Input: part model. Units: mm. Frame: model coordinates. A direction names the side the tool comes from. Round coordinates to 2 decimals unless told otherwise and drop trailing zeros. Order: outer loops, then holes, each group sorted by start corner. A loop starts at its lowest first (then second) coordinate and runs counter-clockwise, first axis right, second up.
Item 1: Cut plane C-C on y = 28.5. Output: boundary loops of the cut face in (x, z).
Item 2: Mould query, pull axis Y, two halves, no side actions, for faces 1 (the flat face through (95.14, 6.44, 33.84)), 2 (the cylindrical face through (9.68, 20.1, 3.13)), 3 (the flat face through (11.43, 7, -3)). Classes: released by +Y, released by -Y, zero draft, split by the parting line, or undercut.
Item 3: First-contact query: pin 1 (1.5 mm diameter, centred on x = 16.5, y = 26, fed in from +Z); pin 2 (6 mm diameter, centred on y = 13.5, z = 16.5, fed in from -X); pin 3 (1.5 mm diameter, centred on y = 8, z = -3, fed in from +X); pin 4 (6.5 mm diameter, centred on x = 51.816, z = -12.7, fed in from +Y). Flat tips, straight axial feed; report the tip coordinate or a pass-through.
Item 4: Cut plane A-A on z = -12.7. Output: boundary loops of the cut face in (x, y), then the cut area to 3 significant figures.
Item 5: Reachability of faces 4 (the flat face through (6, 13.97, -3)), 5 (the flat face through (38.1, 25, -13)), 6 (the flat face through (52, 25.4, -15)) from +Z, -Z, +X, -X, +Y, -Y: full face, straight path, thin tool, end or side. Return the list, or none.
Item 6: Line query: L1, parallel to Y at x = 6, z = 4; L2, parallel to X at y = 25.5, z = -12.5; L3, parallel to X at y = 20.5, z = -13. Output: solid intervals per line, ascending.
```python
from build123d import *

# Parameters (mm, degrees)
SKETCH2_R           = 2.0828
BOSS_EXTRUDE1_DEPTH = 31.75
SKETCH4_W           = 31.75
SKETCH4_H           = 12.7
CUT_EXTRUDE1_DEPTH  = 19.05
SKETCH5_R           = 3.4925
CUT_EXTRUDE2_DEPTH  = 6.35
CUT_EXTRUDE6_DEPTH  = 19.05
CHAMFER5_SIZE       = 12.7
CHAMFER7_SIZE       = 12.7
SKETCH6_R           = 3.4925
CUT_EXTRUDE8_DEPTH  = 25.4
SKETCH15_R          = 3.4925
SKETCH15_R_2        = 2.0828
BOSS_EXTRUDE2_DEPTH = 6.35
SKETCH14_W          = 11.43
SKETCH14_H          = 13.97
CUT_EXTRUDE10_DEPTH = 6.35


with BuildPart() as part:
    # Sketch2 → Boss-Extrude1 (new body)
    with BuildSketch(Plane(origin=(0, 0, 0), x_dir=(1, 0, 0), z_dir=(0, 1, 0))):
        Polygon((-69.85, 6.35), (-76.2, 6.35), (-76.2, 0), (-127, 0), (-73.025, -76.2), (0, 0), (0, 6.35), (-38.1, 6.35), (-38.1, 19.05), (-69.85, 19.05), align=None)
        with Locations(Location((-51.816, 12.7, 0), (0, 0, 270))):
            Circle(SKETCH2_R, mode=Mode.SUBTRACT)
        Polygon((-38.556305928, -12.7), (-69.85, -12.7), (-76.2, -12.7), (-94.65927881, -12.7), (-70.815515335, -46.361783729), align=None, mode=Mode.SUBTRACT)
    extrude(amount=BOSS_EXTRUDE1_DEPTH)

    # Sketch4 → Cut-Extrude1 (cut)
    with BuildSketch(Plane.XZ):
        with Locations((-53.975, -12.7)):
            Rectangle(SKETCH4_W, SKETCH4_H)
    extrude(amount=-CUT_EXTRUDE1_DEPTH, mode=Mode.SUBTRACT)

    # Sketch5 → Cut-Extrude2 (cut)
    with BuildSketch(Plane(origin=(0, 19.05, 0), x_dir=(-1, 0, 0), z_dir=(0, -1, 0))):
        with Locations(Location((51.816, 12.7, 0), (0, 0, 90))):
            Circle(SKETCH5_R)
    extrude(amount=-CUT_EXTRUDE2_DEPTH, mode=Mode.SUBTRACT)

    # Sketch3 → Cut-Extrude6 (cut)
    with BuildSketch(Plane(origin=(0, 31.75, 0), x_dir=(1, 0, 0), z_dir=(0, 1, 0))):
        Polygon((-127, 0), (-73.025, -76.2), (-6.085416667, -6.35), (-23.67573173, -6.35), (-71.552010223, -56.307855819), (-111.436741429, 0), align=None)
    extrude(amount=-CUT_EXTRUDE6_DEPTH, mode=Mode.SUBTRACT)

    # Chamfer5
    chamfer5_edges = [part.edges().sort_by_distance(p)[0] for p in [
        (-39.555208333, 12.7, 41.275),
    ]]
    chamfer(chamfer5_edges, length=CHAMFER5_SIZE - 0.0001)  # a hair under: the kernel refuses the full size

    # Chamfer7
    chamfer7_edges = [part.edges().sort_by_distance(p)[0] for p in [
        (-103.750412518, 12.7, 32.822947033),
    ]]
    chamfer(chamfer7_edges, length=CHAMFER7_SIZE - 0.0001)  # a hair under: the kernel refuses the full size

    # Sketch6 → Cut-Extrude8 (cut)
    with BuildSketch(Plane(origin=(0, 0, -6.35), x_dir=(-1, 0, 0), z_dir=(0, 0, -1))):
        with Locations((6.35, 19.05)):
            Circle(SKETCH6_R)
    extrude(amount=-CUT_EXTRUDE8_DEPTH, mode=Mode.SUBTRACT)

    # Sketch15 → Boss-Extrude2 (add)
    with BuildSketch(Plane(origin=(0, 0, -6.35), x_dir=(-1, 0, 0), z_dir=(0, 0, -1))):
        with Locations((6.35, 19.05)):
            Circle(SKETCH15_R)
        with Locations((6.35, 19.05)):
            Circle(SKETCH15_R_2, mode=Mode.SUBTRACT)
    extrude(amount=-BOSS_EXTRUDE2_DEPTH)

    # Sketch14 → Cut-Extrude10 (cut)
    with BuildSketch(Plane(origin=(0, 0, -6.35), x_dir=(-1, 0, 0), z_dir=(0, 0, -1))):
        with Locations((5.715, 6.985)):
            Rectangle(SKETCH14_W, SKETCH14_H)
    extrude(amount=-CUT_EXTRUDE10_DEPTH, mode=Mode.SUBTRACT)


with BuildPart() as body_2:
    # Mirror1: mirrored copy
    add(part.part.mirror(Plane(origin=(0, 31.75, 0), x_dir=(0, 0, 1), z_dir=(-1, 0, 0))))


solid = body_2.part
```
From the geometry:
1. outline: (0, -6.35) - (38.1, -6.35) - (38.1, -19.05) - (69.85, -19.05) - (69.85, -6.35) - (76.2, -6.35) - (76.2, 0) - (111.44, 0) - (71.55, 56.31) - (23.68, 6.35) - (6.09, 6.35) - (0, 0) - close; hole (38.56, 12.7) - (94.66, 12.7) - (70.82, 46.36) - close; hole circle Ø4.17 at (51.82, -12.7)
2. face 1: released by +Y
2. face 2: undercut
2. face 3: zero draft
3. pin 1: stops at z = 6.35
3. pin 2: stops at x = 29.46
3. pin 3: stops at x = 76.2
3. pin 4: stops at y = 31.75
4. outline: (38.1, 19.05) - (48.32, 19.05) - (48.32, 25.4) - (49.73, 25.4) - (49.73, 31.75) - (38.1, 31.75) - close; (53.9, 25.4) - (55.31, 25.4) - (55.31, 19.05) - (69.85, 19.05) - (69.85, 31.75) - (53.9, 31.75) - close
4. area: 332 mm2
5. face 4: -Z, -X, -Y
5. face 5: -Z, -X, +Y, -Y
5. face 6: -Y
6. L1: y = 0 to 15.58, 22.52 to 31.75
6. L2: x = 38.1 to 49.74, 53.89 to 69.85
6. L3: x = 38.1 to 48.34, 55.3 to 69.85
